from build123d import *
from build123d.topology import SkipClean

# Parameters (mm, degrees)
SKETCH1_W           = 53.975
SKETCH1_H           = 25.4
SKETCH1_R           = 3.175
SKETCH1_R_2         = 9.525
BOSS_EXTRUDE2_DEPTH = 6.35
SKETCH1_5_R         = 9.525
SKETCH1_5_R_2       = 6.35
BOSS_EXTRUDE3_DEPTH = 2.778125
FILLET1_R           = 1.27
CUT_EXTRUDE1_DEPTH  = 60.989858518


# Read off the part's stored shape, not the designer's step: Cut-Revolve3
with BuildPart() as part:
    # Sketch1 → Boss-Extrude2 (new body)
    # profile 1 of 2: a face of its own
    with SkipClean():  # the faces are left unmerged after this step: merging them gives an invalid solid
        with BuildSketch(Plane.XY):
            with Locations((26.9875, -12.7)):
                Rectangle(SKETCH1_W, SKETCH1_H)
            with Locations((22.225, -12.7)):
                Circle(SKETCH1_R, mode=Mode.SUBTRACT)
            with Locations((9.525, -12.7)):
                Circle(SKETCH1_R, mode=Mode.SUBTRACT)
            with Locations((41.275, -12.7)):
                Circle(SKETCH1_R_2, mode=Mode.SUBTRACT)
        # profile 2 of 2: a face of its own
        with BuildSketch(Plane.XY):
            with BuildLine():
                Line((53.975, -12.7), (50.8, -12.7))
                ThreePointArc((50.8, -12.7), (41.275, -22.225), (31.75, -12.7))
                Line((31.75, -12.7), (25.4, -12.7))
                ThreePointArc((25.4, -12.7), (22.225, -15.875), (19.05, -12.7))
                Line((19.05, -12.7), (12.7, -12.7))
                ThreePointArc((12.7, -12.7), (9.525, -15.875), (6.35, -12.7))
                Line((6.35, -12.7), (0, -12.7))
                Line((0, -12.7), (0, -25.4))
                Line((0, -25.4), (53.975, -25.4))
                Line((53.975, -25.4), (53.975, -12.7))
            make_face()
        extrude(amount=BOSS_EXTRUDE2_DEPTH)
    add(part.part.scale(1), mode=Mode.REPLACE)  # the faces are merged on a copy

    # Sketch1_5 → Boss-Extrude3 (add)
    # profile 1 of 3: a face of its own
    with BuildSketch(Plane.XY):
        with Locations((41.275, -12.7)):
            Circle(SKETCH1_5_R)
        with Locations((41.275, -12.7)):
            Circle(SKETCH1_5_R_2, mode=Mode.SUBTRACT)
    # profile 2 of 3: a face of its own
    with BuildSketch(Plane.XY):
        with BuildLine():
            ThreePointArc((34.925, -12.7), (41.275, -6.35), (47.625, -12.7))
            Line((47.625, -12.7), (50.8, -12.7))
            ThreePointArc((50.8, -12.7), (41.275, -3.175), (31.75, -12.7))
            Line((31.75, -12.7), (34.925, -12.7))
        make_face()
    # profile 3 of 3: a face of its own
    with BuildSketch(Plane.XY):
        with BuildLine():
            Line((50.8, -12.7), (47.625, -12.7))
            ThreePointArc((47.625, -12.7), (41.275, -19.05), (34.925, -12.7))
            Line((34.925, -12.7), (31.75, -12.7))
            ThreePointArc((31.75, -12.7), (41.275, -22.225), (50.8, -12.7))
        make_face()
    extrude(amount=BOSS_EXTRUDE3_DEPTH)

    # Fillet1
    fillet1_edges = [part.edges().sort_by_distance(p)[0] for p in [
        (0, 0, 3.175),
        (53.975, 0, 3.175),
        (53.975, -25.4, 3.175),
        (0, -25.4, 3.175),
    ]]
    fillet(fillet1_edges, radius=FILLET1_R)

    # Sketch2 → Cut-Extrude1 (cut, through all)
    with BuildSketch(Plane.XY.offset(6.35)):
        with BuildLine():
            ThreePointArc((41.275, 0), (50.255256121, -3.719743879), (53.975, -12.7))
            Line((53.975, -12.7), (53.975, -1.27))
            ThreePointArc((53.975, -1.27), (53.603025612, -0.371974388), (52.705, 0))
            Line((52.705, 0), (41.275, 0))
        make_face()
        with BuildLine():
            Line((41.275, -25.4), (52.705, -25.4))
            ThreePointArc((52.705, -25.4), (53.603025612, -25.028025612), (53.975, -24.13))
            Line((53.975, -24.13), (53.975, -12.7))
            ThreePointArc((53.975, -12.7), (50.255256121, -21.680256121), (41.275, -25.4))
        make_face()
    extrude(amount=-CUT_EXTRUDE1_DEPTH, mode=Mode.SUBTRACT)

    # Cut-Revolve3 outline → Cut-Revolve3 (revolve, cut)
    with BuildSketch(Plane(origin=(41.275, -12.7, 0), x_dir=(1, 0, 0), z_dir=(0, -1, 0))):
        Polygon((6.35, 0), (8.06821119, 0), (6.831310248, 2.778125), (6.35, 2.778125), align=None)
    revolve(axis=Axis((41.275, -12.7, 0), (0, 0, 1)), mode=Mode.SUBTRACT)


solid = part.part
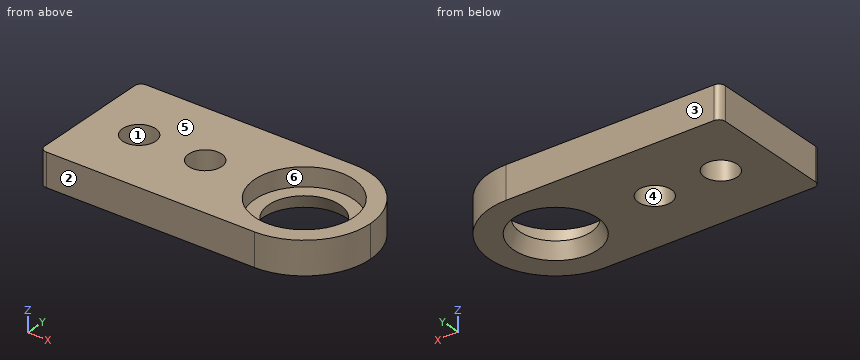
For this review, take the finished solid that the model builds, in its own axes (mm). Face numbers are marked on the shaded views. A direction names the side the tool comes from. Round coordinates to 2 decimals unless told otherwise and drop trailing zeros. Write each loop counter-clockwise with the first axis right and the second up, starting at its lowest first coordinate (ties: lowest second). Pieces come first, ordered by that corner, then holes. Notation, with made-up numbers: (11, 36.5) -> (27, 36.5) arc R26 ccw to (27, 53.5) -> close; hole circle Ø11 at (7, -7). An arc over 180 degrees is marked (long way). Put each result on its own line as item: value.
Q1. To check wall thickness, follow L1, parallel to X at y = -22.5, z = 5.25; L2, parallel to X at y = -5.25, z = 6; L3, parallel to Y at x = 24, z = 3. State the ranges of each line that lie inside material, in increasing order. Write a range as [from, to].
Determined:
L1: x = [0, 49.35]
L2: x = [0, 35.34], [47.21, 51.56]
L3: y = [-25.4, -15.33], [-10.07, 0]
Q2. The part is to be moulded in two halves that separate along Y. For the marked faces 1, 2, 3 and 4, say which applies: released by +Y, released by -Y, zero draft, split by the parting line, or undercut.
Determined:
face 1: undercut
face 2: released by -Y
face 3: released by +Y
face 4: undercut
Q3. Clearance check with a flat-ended pin moving along its axis: pin 1 Ø5 at (x, y) = (9.525, -12.7) entering from -Z. State where the tip first meets the part, or that it passes through.
Determined:
pin 1: passes through
Q4. Consider section A-A on z = 1.5. State the section outline as (x, y) points (3 decimals), and give its area (3 significant figures).
Determined:
outline: (0, -24.13) arc R1.27 ccw to (1.27, -25.4) -> (41.275, -25.4) arc R12.7 ccw to (41.275, 0) -> (1.27, 0) arc R1.27 ccw to (0, -1.27) -> close; hole circle Ø6.35 at (9.525, -12.7); hole circle Ø6.35 at (22.225, -12.7); hole circle Ø14.801 at (41.275, -12.7)
area: 1,070 mm^2
Q5. Consider section B-B on z = 4.25. State the section outline as (x, y) points (3 decimals), and give its area (3 significant figures).
Determined:
outline: (0, -24.13) arc R1.27 ccw to (1.27, -25.4) -> (41.275, -25.4) arc R12.7 ccw to (41.275, 0) -> (1.27, 0) arc R1.27 ccw to (0, -1.27) -> close; hole circle Ø6.35 at (9.525, -12.7); hole circle Ø6.35 at (22.225, -12.7); hole circle Ø19.05 at (41.275, -12.7)
area: 953 mm^2
Q6. Machinability: for the marked faces 5 and 6, which of the approach directions +Z, -Z, +X, -X, +Y, -Y give a long, thin tool a straight path to every point of the face, cutting with its end or side? Answer none if there is none.
Determined:
face 5: +Z, +X, -X, +Y, -Y
face 6: +Z
